```python
from build123d import *

# Parameters (mm, degrees)
SKETCH1_W           = 21.5
SKETCH1_H           = 14
BOSS_EXTRUDE1_DEPTH = 3.5


with BuildPart() as part:
    # Sketch1 → Boss-Extrude1 (new body)
    with BuildSketch(Plane(origin=(0, 0, 0), x_dir=(1, 0, 0), z_dir=(0, 1, 0))):
        Polygon((40, 16.568542495), (16.568542495, 40), (-16.568542495, 40), (-40, 16.568542495), (-40, -16.568542495), (-16.568542495, -40), (16.568542495, -40), (40, -16.568542495), align=None)
        Rectangle(SKETCH1_W, SKETCH1_H, mode=Mode.SUBTRACT)
    extrude(amount=BOSS_EXTRUDE1_DEPTH)


solid = part.part
```
For this review, take the finished solid that the model builds, in its own axes (mm). A direction names the side the tool comes from. Round coordinates to 2 decimals unless told otherwise and drop trailing zeros. Write each loop counter-clockwise with the first axis right and the second up, starting at its lowest first coordinate (ties: lowest second). Pieces come first, ordered by that corner, then holes. Notation, with made-up numbers: (10.25, 32.5) - (53.25, 32.5) arc R25 cw to (53.25, 51.5) - close; hole circle Ø10 at (74, 33). An arc over 180 degrees is marked (long way). Answer as CSV lines item,"result". Start each with the question number.
(1) For pin 1 (1 mm diameter, centred on y = 1, z = -29, fed in from -X), flat-tipped, find the tip position at first contact; note if it passes through.
(2) Add section B-B, the plane x = 7. State the section outline as (y, z) points.
(3) Add section A-A, the plane z = -1. State the section outline as (x, y) points.
(4) For line 1 (X direction, y = 1.2, z = 4.5); line 2 (Z direction, x = 19, y = 1.4); line 3 (X direction, y = 0.4, z = 24), list the stretches that pass through material, from the lowest coordinate up.
(5) Add section C-C, the plane y = 2.25. State the section outline as (x, z) points.
(6) Mouldability with a two-part tool opening along X and no side actions: class faces 3 (the flat face through (28.12, 1.73, 28.45)), 4 (the flat face through (0, 2, 7)), 5 (the flat face through (-28.45, 1.73, 28.12)) as +X half, -X half, draft (parallel to the pull), parting line (faces both ways), or undercut.
(7) Machinability: for faces 1 (the flat face through (10.75, 2, 0)), 2 (the flat face through (0, 2, -40)), which of the approach directions +Z, -Z, +X, -X, +Y, -Y give a long, thin tool a straight path to every point of the face, cutting with its end or side? Answer none if there is none.
(8) Add section D-D, the plane z = 23.5. State the section outline as (x, y) points.
From the geometry:
1,pin 1,"stops at x = -28.07"
2,outline,"(0, -40) - (3.5, -40) - (3.5, -7) - (0, -7) - close; (0, 7) - (3.5, 7) - (3.5, 40) - (0, 40) - close"
3,outline,"(-40, 0) - (-10.75, 0) - (-10.75, 3.5) - (-40, 3.5) - close; (10.75, 0) - (40, 0) - (40, 3.5) - (10.75, 3.5) - close"
4,line 1,"x = -40 to -10.75, 10.75 to 40"
4,line 2,"z = -37.57 to 37.57"
4,line 3,"x = -32.57 to 32.57"
5,outline,"(-40, -16.57) - (-16.57, -40) - (16.57, -40) - (40, -16.57) - (40, 16.57) - (16.57, 40) - (-16.57, 40) - (-40, 16.57) - close; hole (-10.75, -7) - (10.75, -7) - (10.75, 7) - (-10.75, 7) - close"
6,face 3,"+X half"
6,face 4,"undercut"
6,face 5,"-X half"
7,face 1,"+Y, -Y"
7,face 2,"-Z, +X, -X, +Y, -Y"
8,outline,"(-33.07, 0) - (33.07, 0) - (33.07, 3.5) - (-33.07, 3.5) - close"
